For this review, take the finished solid that the model builds, in its own axes (mm). Face numbers are marked on the shaded views. Coordinates: 2 decimals unless noted, no trailing zeros. Loops run counter-clockwise (first coordinate to the right, second up) from the corner with the lowest first, then second, coordinate; pieces in that order, holes last. Notation, with made-up numbers: (-32.75, 41.25) - (22.25, 41.25) arc R13 cw to (22.25, 59.25) - close; hole circle Ø1 at (-4, -1.75). An arc over 180 degrees is marked (long way). Answer as a JSON object with one key per item and string values. Group by question number.
Item 1: We need section C-C (x = -5.5). Give the boundary of the cut face in (y, z).
Item 2: Mouldability with a two-part tool opening along Z and no side actions: class the marked faces 1 and 2 as released by +Z, released by -Z, zero draft, split by the parting line, or undercut.
Item 3: To check wall thickness, follow line 1 (X direction, y = -1, z = 80); line 2 (Z direction, x = -5, y = 1.35); line 3 (Z direction, x = 5, y = 0). State the ranges of each line that lie inside material, in increasing order.
Item 4: We need section A-A (x = 0). Give the boundary of the cut face in (y, z).
Item 5: We need section D-D (z = 57). Give the boundary of the cut face in (x, y), then the cut area to 3 significant figures.
Item 6: Clearance check with flat-ended pins moving along their axes: pin 1 (4 mm diameter, centred on x = -6, y = 1, fed in from -Z); pin 2 (4 mm diameter, centred on x = -5, z = 80, fed in from +Y); pin 3 (8 mm diameter, centred on x = -5.5, y = -11, fed in from -Z). State where each tip first meets the part, or that it passes through.
Item 7: We need section B-B (z = 80). Give the boundary of the cut face in (x, y).
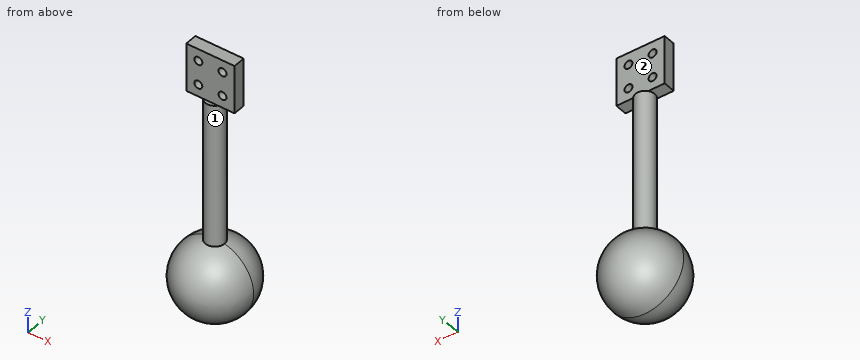
from build123d import *

# Parameters (mm, degrees)
SKETCH1_3_R              = 4
BOSS_EXTRUDE1_DEPTH      = 75
SKETCH2_R                = 1.65
BOSS_EXTRUDE2_DEPTH      = 2.5
BOSS_EXTRUDE2_DEPTH_BACK = 2.5


with BuildPart() as part:
    # Sketch1 one side → Revolve7 (revolve)
    with BuildSketch(Plane.XY):
        with BuildLine():
            ThreePointArc((0, -16), (11.313708499, -11.313708499), (16, 0))
            ThreePointArc((16, 0), (11.313708499, 11.313708499), (0, 16))
            Line((0, 16), (0, 4))
            ThreePointArc((0, 4), (2.828427125, 2.828427125), (4, 0))
            ThreePointArc((4, 0), (2.828427125, -2.828427125), (0, -4))
            Line((0, -4), (0, -16))
        make_face()
    revolve(axis=Axis((0, 16, 0), (0, -1, 0)))

    # Sketch1_3 → Boss-Extrude1 (add)
    with BuildSketch(Plane.XY):
        Circle(SKETCH1_3_R)
    extrude(amount=BOSS_EXTRUDE1_DEPTH)

    # Sketch2 → Boss-Extrude2 (add, two sides)
    with BuildSketch(Plane(origin=(0, 0, 0), x_dir=(1, 0, 0), z_dir=(0, 1, 0))) as boss_extrude2_sk:
        Polygon((10, -85), (-10, -85), (-10, -95), (0, -95), (10, -95), align=None)
        with Locations((-5, -90)):
            Circle(SKETCH2_R, mode=Mode.SUBTRACT)
        with Locations((5, -90)):
            Circle(SKETCH2_R, mode=Mode.SUBTRACT)
        Polygon((10, -75), (0, -75), (-10, -75), (-10, -85), (10, -85), align=None)
        with Locations((-5, -80)):
            Circle(SKETCH2_R, mode=Mode.SUBTRACT)
        with Locations((5, -80)):
            Circle(SKETCH2_R, mode=Mode.SUBTRACT)
    extrude(amount=BOSS_EXTRUDE2_DEPTH)
    extrude(boss_extrude2_sk.sketch, amount=-BOSS_EXTRUDE2_DEPTH_BACK)


solid = part.part
Check sheet entries:
{
 "1": {"outline": "circle Ø30.05 at (0, 0); (-2.5, 75) - (2.5, 75) - (2.5, 78.43) - (-2.5, 78.43) - close; (-2.5, 81.57) - (2.5, 81.57) - (2.5, 88.43) - (-2.5, 88.43) - close; (-2.5, 91.57) - (2.5, 91.57) - (2.5, 95) - (-2.5, 95) - close"},
 "2": {"face 1": "undercut", "face 2": "zero draft"},
 "3": {"line 1": "x = -10 to -6.65, -3.35 to 3.35, 6.65 to 10", "line 2": "z = -15.14 to 15.14, 75 to 78.35, 81.65 to 88.35, 91.65 to 95", "line 3": "z = -15.2 to 15.2, 75 to 78.35, 81.65 to 88.35, 91.65 to 95"},
 "4": {"outline": "(-4, 15.49) arc R16 ccw (long way) to (4, 15.49) - (4, 75) - (2.5, 75) - (2.5, 95) - (-2.5, 95) - (-2.5, 75) - (-4, 75) - close; hole (-4, 0) arc R4 ccw to (4, 0) - close"},
 "5": {"outline": "circle Ø8 at (0, 0)", "area": "50.3 mm2"},
 "6": {"pin 1": "stops at z = -15.47", "pin 2": "stops at y = 2.5", "pin 3": "stops at z = -13.68"},
 "7": {"outline": "(-10, -2.5) - (-6.65, -2.5) - (-6.65, 2.5) - (-10, 2.5) - close; (-3.35, -2.5) - (3.35, -2.5) - (3.35, 2.5) - (-3.35, 2.5) - close; (6.65, -2.5) - (10, -2.5) - (10, 2.5) - (6.65, 2.5) - close"}
}
